from build123d import *

# Parameters (mm, degrees)
SALIENTE_EXTRUIR1_DEPTH             = 47
CROQUIS2_W                          = 6.2
CROQUIS2_H                          = 6.535373831
CORTAR_EXTRUIR1_DEPTH               = 17.248076809
CROQUIS3_W                          = 10.5
CROQUIS3_H                          = 14
CORTAR_EXTRUIR2_DEPTH               = 17.248076809
NGULO_DE_SALIDA1_ANGLE              = 18.434948823
NGULO_DE_SALIDA2_ANGLE              = -18.434948823
TALADRO1_D                          = 5.1
TALADRO1_DEPTH                      = 8
TALADRO1_CBORE_D                    = 10.5
TALADRO1_CBORE_DEPTH                = 6
CROQUIS6_W                          = 1.9
CROQUIS6_H                          = 7.15
DI_METRO_DE_TALADRO_3_8_3_8_2_D     = 3.8
DI_METRO_DE_TALADRO_3_8_3_8_2_DEPTH = 7.15


with BuildPart() as part:
    # Croquis1 → Saliente-Extruir1 (new body)
    with BuildSketch(Plane(origin=(0, 0, 117.639), x_dir=(-1, 0, 0), z_dir=(0, 0, -1))):
        with BuildLine():
            Line((-6.25, 309.279690095), (6.25, 309.279690095))
            ThreePointArc((6.25, 309.279690095), (10.25, 317.403728499), (6.25, 325.527766904))
            Line((6.25, 325.527766904), (-6.25, 325.527766904))
            ThreePointArc((-6.25, 325.527766904), (-10.25, 317.403728499), (-6.25, 309.279690095))
        make_face()
    extrude(amount=-SALIENTE_EXTRUIR1_DEPTH)

    # Croquis2 → Cortar-Extruir1 (cut, through all)
    with BuildSketch(Plane(origin=(0, 325.527766904, 0), x_dir=(-1, 0, 0), z_dir=(0, 1, 0))):
        with Locations((0, 129.060696737)):
            Rectangle(CROQUIS2_W, CROQUIS2_H)
    extrude(amount=-CORTAR_EXTRUIR1_DEPTH, mode=Mode.SUBTRACT)

    # Croquis3 → Cortar-Extruir2 (cut, through all)
    with BuildSketch(Plane.XZ.offset(-309.279690095)):
        with Locations((0, 149.639)):
            Rectangle(CROQUIS3_W, CROQUIS3_H)
    extrude(amount=-CORTAR_EXTRUIR2_DEPTH, mode=Mode.SUBTRACT)

    # Ángulo de salida1
    ngulo_de_salida1_faces = [part.faces().sort_by_distance(p)[0] for p in [
        (0, 317.403728499, 125.793009821),
    ]]
    draft(ngulo_de_salida1_faces, Plane(origin=(6.25, 309.279690095, 164.639), x_dir=(0, 0, -1), z_dir=(0, -1, 0)), NGULO_DE_SALIDA1_ANGLE)

    # Ángulo de salida2
    ngulo_de_salida2_faces = [part.faces().sort_by_distance(p)[0] for p in [
        (0, 317.403728499, 132.328383652),
    ]]
    draft(ngulo_de_salida2_faces, Plane(origin=(6.25, 309.279690095, 164.639), x_dir=(0, 0, -1), z_dir=(0, -1, 0)), NGULO_DE_SALIDA2_ANGLE)

    # Taladro1
    with Locations(Plane(origin=(0, 0, 156.639), x_dir=(-1, 0, 0), z_dir=(0, 0, -1))):
        with Locations((0, 317.403728499)):
            CounterBoreHole(TALADRO1_D / 2, TALADRO1_CBORE_D / 2, TALADRO1_CBORE_DEPTH, depth=TALADRO1_DEPTH)

    # Croquis6 → Diámetro de taladro Ø3.8 (3.8)1 (revolve, cut)
    with BuildSketch(Plane(origin=(3.1, 317.403728499, 131.768709538), x_dir=(0, 0, 1), z_dir=(0, 1, 0))):
        with Locations((0.95, 3.575)):
            Rectangle(CROQUIS6_W, CROQUIS6_H)
    revolve(axis=Axis((-3.25, 317.403728499, 131.768709538), (1, 0, 0)), mode=Mode.SUBTRACT)

    # Diámetro de taladro Ø3.8 (3.8)2
    with Locations(Plane(origin=(-3.1, 0, 0), x_dir=(0, 0, -1), z_dir=(1, 0, 0))):
        with Locations((-131.768709538, 317.403728499)):
            Hole(DI_METRO_DE_TALADRO_3_8_3_8_2_D / 2, depth=DI_METRO_DE_TALADRO_3_8_3_8_2_DEPTH)


solid = part.part
Check sheet for the modelled part. Datum: model origin and axes. Units: mm. A direction names the side the tool comes from. Give positions to 0.01 mm unless a question says otherwise; leave off trailing zeros. Write each loop counter-clockwise with the first axis right and the second up, starting at its lowest first coordinate (ties: lowest second). Pieces come first, ordered by that corner, then holes. Notation, with made-up numbers: (-25.75, 11) -> (30.25, 11) arc R34 ccw to (30.25, 45) -> close; hole circle Ø11 at (7.25, 30). An arc over 180 degrees is marked (long way). Write item = value, one per line.
Item 1: Sectioned sample at B-B on y = 321.25. Record the boundary of the cut face in (x, z).
Output:
outline = (-9.5, 117.64) -> (9.5, 117.64) -> (9.5, 164.64) -> (-9.5, 164.64) -> close; hole (-5.25, 142.64) -> (5.25, 142.64) -> (5.25, 156.64) -> (3.57, 156.64) -> (3.57, 162.64) -> (-3.57, 162.64) -> (-3.57, 156.64) -> (-5.25, 156.64) -> close; hole (-3.1, 129.78) -> (3.1, 129.78) -> (3.1, 136.32) -> (-3.1, 136.32) -> close
Item 2: Sectioned sample at D-D on z = 162. Record the boundary of the cut face in (x, y), and give its area (3 significant figures).
Output:
outline = (-6.25, 309.28) -> (6.25, 309.28) arc R10.25 ccw to (6.25, 325.53) -> (-6.25, 325.53) arc R10.25 ccw to start; hole circle Ø10.5 at (0, 317.4)
area = 207 mm^2
Item 3: Gauge pin test, flat ends, axial feed: pin 1 (4 mm diameter, centred on x = 0, y = 317.4, fed in from +Z); pin 2 (4 mm diameter, centred on y = 322, z = 123.5, fed in from +X); pin 3 (7 mm diameter, centred on y = 316, z = 147, fed in from -X); pin 4 (6 mm diameter, centred on y = 313.5, z = 129, fed in from +X). Record the tip position at first contact, or that the pin passes through.
Output:
pin_1 = 142.64
pin_2 = 9.92
pin_3 = -10.25
pin_4 = 10.21
Item 4: Sectioned sample at A-A on x = 0. Record the boundary of the cut face in (y, z), and give its area (3 significant figures).
Output:
outline = (309.28, 117.64) -> (325.53, 117.64) -> (325.53, 131.21) -> (309.28, 125.79) -> close; (309.28, 132.33) -> (325.53, 137.74) -> (325.53, 142.64) -> (309.28, 142.64) -> close; (309.28, 156.64) -> (312.15, 156.64) -> (312.15, 162.64) -> (314.85, 162.64) -> (314.85, 164.64) -> (309.28, 164.64) -> close; (319.95, 162.64) -> (322.65, 162.64) -> (322.65, 156.64) -> (325.53, 156.64) -> (325.53, 164.64) -> (319.95, 164.64) -> close
area = 357 mm^2
Item 5: Scan lines: probe 1 along Z at (x, y) = (3.25, 318.5); probe 2 along Z at (x, y) = (0.5, 321); probe 3 along Y at (x, z) = (0, 163.4). Record each from-to range of solid material in increasing order. Write a range as from..to.
Output:
probe_1 = 117.64..130.22, 133.32..142.64, 162.64..164.64
probe_2 = 117.64..129.7, 136.24..142.64, 162.64..164.64
probe_3 = 309.28..314.85, 319.95..325.53
Item 6: Release check for a two-part mould opening along Y. For faces 6 (the cylindrical face through (-6.73, 315.72, 132.65)), 7 (the cylindrical face through (6.73, 315.8, 132.79)), 8 (the flat face through (0, 309.28, 136)), 9 (the flat face through (0, 323, 156.639)) record: +Y half, -Y half, draft (parallel to the pull), parting line (faces both ways), or undercut.
Output:
face_6 = undercut
face_7 = undercut
face_8 = -Y half
face_9 = draft
Item 7: Tool access check on faces 1 (the cylindrical face through (-10.25, 317.27, 140.81)), 2 (the flat face through (-5.25, 317, 150)), 3 (the flat face through (-1, 320, 162.639)), 4 (the cylindrical face through (1.177, 315.141, 163.653)), 5 (the flat face through (0.043, 317.517, 135.074)). Record the directions out of +Z, -Z, +X, -X, +Y, -Y that give a thin tool (end or side, any length) a straight path to the whole face; none if there is none.
Output:
face_1 = +Z, -Z, -X
face_2 = +Y, -Y
face_3 = none
face_4 = +Z
face_5 = +Y
Item 8: Sectioned sample at C-C on z = 133. Record the boundary of the cut face in (x, y).
Output:
outline = (-10.15, 315.96) arc R10.25 ccw to (-6.25, 309.28) -> (6.25, 309.28) arc R10.25 ccw to (10.15, 315.96) -> (3.1, 315.96) -> (3.1, 311.29) -> (-3.1, 311.29) -> (-3.1, 315.96) -> close; (-10.15, 318.85) -> (-3.1, 318.85) -> (-3.1, 325.53) -> (-6.25, 325.53) arc R10.25 ccw to start; (3.1, 318.85) -> (10.15, 318.85) arc R10.25 ccw to (6.25, 325.53) -> (3.1, 325.53) -> close
